Autodesk Inventor part; units mm, degrees
ref_plane "YZ Plane" through (0, 0, 0) normal (1, 0, 0) x (0, 1, 0)
ref_plane "XZ Plane" through (0, 0, 0) normal (0, 1, 0) x (-1, 0, 0)
ref_plane "XY Plane" through (0, 0, 0) normal (0, 0, 1) x (1, 0, 0)
sketch "Sketch1" plane through (0, 0, 0) normal (0, 1, 0) x (-1, 0, 0)
  line L0 (140.4432, 454.8476) -> (-259.5568, 454.8476)
  line L1 (-259.5568, 454.8476) -> (-259.5568, -245.1524)
  line L2 (-259.5568, -245.1524) -> (140.4432, -245.1524)
  line L3 (140.4432, -245.1524) -> (140.4432, 454.8476)
  point P0 (0, 0)
  dimension "d0" = 700
  dimension "d1" = 400
extrude "Extrusion1" add sketch "Sketch1" along normal blind 8
sketch "Sketch2" plane through (0, 8, 0) normal (0, 1, 0) x (1, 0, 0)
  line L0 (-140.4432, 245.1524) -> (-140.4432, -454.8476)
  line L1 (-140.4432, -454.8476) -> (-89.6432, -454.8476)
  line L2 (-89.6432, -454.8476) -> (-89.6432, -404.0476)
  line L3 (-89.6432, -404.0476) -> (-140.4432, -404.0476)
  line L4 (-140.4432, -404.0476) -> (-140.4432, -454.8476)
  line L5 (259.5568, -454.8476) -> (259.5568, 245.1524)
  line L6 (259.5568, -454.8476) -> (208.7568, -454.8476)
  line L7 (208.7568, -454.8476) -> (208.7568, -404.0476)
  line L8 (208.7568, -404.0476) -> (259.5568, -404.0476)
  line L9 (259.5568, -404.0476) -> (259.5568, -454.8476)
  line L10 (259.5568, 245.1524) -> (208.7568, 245.1524)
  line L11 (208.7568, 245.1524) -> (208.7568, 194.3524)
  line L12 (208.7568, 194.3524) -> (259.5568, 194.3524)
  line L13 (259.5568, 194.3524) -> (259.5568, 245.1524)
  line L14 (-140.4432, 245.1524) -> (-89.6432, 245.1524)
  line L15 (-89.6432, 245.1524) -> (-89.6432, 194.3524)
  line L16 (-89.6432, 194.3524) -> (-140.4432, 194.3524)
  line L17 (-140.4432, 194.3524) -> (-140.4432, 245.1524)
  point P0 (0, 0)
  point P1 (259.5568, -404.0476)
  dimension "d4" = 50.8
  dimension "d5" = 50.8
  dimension "d6" = 50.8
  dimension "d7" = 50.8
  dimension "d8" = 50.8
  dimension "d9" = 50.8
  dimension "d10" = 50.8
extrude "Extrusion2" add sketch "Sketch2" along normal blind 101.6
properties part number "board" material "Wood (Birch)"
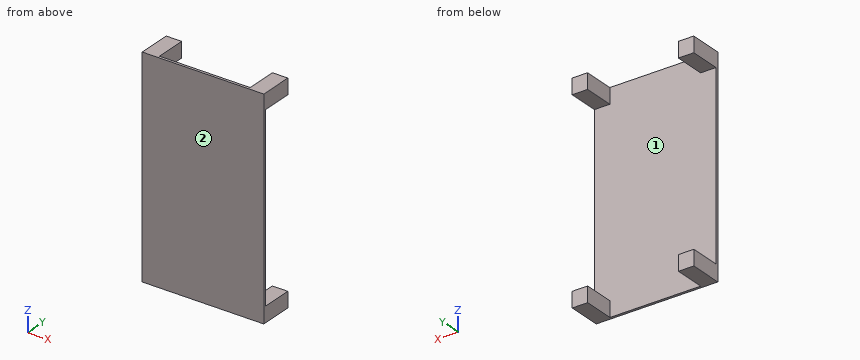
Work out the finished part from the listing and answer in its coordinate system (mm). Face numbers are marked on the shaded views. Coordinates: 2 decimals unless noted, no trailing zeros. Loops run counter-clockwise (first coordinate to the right, second up) from the corner with the lowest first, then second, coordinate; pieces in that order, holes last. Notation, with made-up numbers: M 3,8 L 13,8 A15 cw 13,13 Z; hole C 18.25,34 d2. An arc over 180 degrees is marked long. Use CSV: the item, a comma, the result in double quotes. Start each with the question number.
(1) Find section B-B, the plane x = 231.5. Give the vertices of the cut face in (y, z), then the cut area to 3 significant figures.
(2) Find section C-C, the plane z = 319. Give the vertices of the cut face in (x, y).
(3) Consider line 1 (Z direction, x = 241.5, y = 70); line 2 (Y direction, x = -37, z = 105.5). Determine where each line is inside the solid, lowest interval first.
(4) Find section D-D, the plane x = 98.5. Give the vertices of the cut face in (y, z), then the cut area to 3 significant figures.
(5) For a pull along Z with two mould halves and no side action, classify the marked faces 1 and 2 as +Z half, -Z half, draft (parallel to the pull), parting line (faces both ways), or undercut.
(6) Given pin 1 Ø8 at (x, z) = (-2.5, 184) entering from +Y; pin 2 Ø5 at (x, z) = (73.5, 101.5) entering from -Y, each flat-ended and moving along its own axis, determine where each tip first touches the part or whether it passes through.
(7) Find section A-A, the plane y = 81.5. Give the vertices of the cut face in (x, z), then the cut area to 3 significant figures.
Recorded:
1,outline,"M 0,-245.15 L 109.6,-245.15 L 109.6,-194.35 L 8,-194.35 L 8,404.05 L 109.6,404.05 L 109.6,454.85 L 0,454.85 Z"
1,area,"15,900 mm^2"
2,outline,"M -140.44,0 L 259.56,0 L 259.56,8 L -140.44,8 Z"
3,line 1,"z = -245.15 to -194.35, 404.05 to 454.85"
3,line 2,"y = 0 to 8"
4,outline,"M 0,-245.15 L 8,-245.15 L 8,454.85 L 0,454.85 Z"
4,area,"5,600 mm^2"
5,face 1,"undercut"
5,face 2,"draft"
6,pin 1,"stops at y = 8"
6,pin 2,"stops at y = 0"
7,outline,"M -140.44,-245.15 L -89.64,-245.15 L -89.64,-194.35 L -140.44,-194.35 Z; M -140.44,404.05 L -89.64,404.05 L -89.64,454.85 L -140.44,454.85 Z; M 208.76,-245.15 L 259.56,-245.15 L 259.56,-194.35 L 208.76,-194.35 Z; M 208.76,404.05 L 259.56,404.05 L 259.56,454.85 L 208.76,454.85 Z"
7,area,"10,300 mm^2"
